Here's how the part is built. I have some questions about the finished solid (model axes, mm). A direction names the side the tool comes from. Round coordinates to 2 decimals unless told otherwise and drop trailing zeros. Write each loop counter-clockwise with the first axis right and the second up, starting at its lowest first coordinate (ties: lowest second). Pieces come first, ordered by that corner, then holes. Notation, with made-up numbers: (-5.5, -11.5) -> (22.5, -11.5) arc R21 cw to (22.5, 3.5) -> close; hole circle Ø4 at (89, -30.75). An arc over 180 degrees is marked (long way). Put each result on its own line as item: value. Start each with the question number.
1) I want a section at A-A, the plane y = 2.4. List the corners of the cut face in (x, z) for me.
2) Will these pins go through, and if not, where does the flat tip stop? P1, Ø0.6, axis at x = 1.5, z = -2, coming from the +Y side; P2, Ø1.4, axis at y = 1.5, z = -3, coming from the -X side; P3, Ø0.9, axis at x = -1.5, z = -6.1, coming from the -Y side; P4, Ø1.7, axis at x = -1.5, z = -2.1, coming from the -Y side.
3) If I drill on line 1 along Z through (x, y) = (-1.5, 1.05); line 2 along X through (y, z) = (1.2, -2.5); line 3 along X through (y, z) = (1.25, -2.75), over which ranges is the centre line in solid material (lowest first)? Write a range as [from, to].
4) I want a section at C-C, the plane z = -6.5. List the corners of the cut face in (x, y) for me, then the cut area to 3 significant figures.
5) I want a section at B-B, the plane x = 0.75. List the corners of the cut face in (y, z) for me.
6) We'd pull the mould along X, two halves only. Please class faces 4 (the flat face through (1, 1.65, -2)), 5 (the flat face through (-6.2, 1, -4)), 6 (the flat face through (-7.53, 1.37, -3.97)): released by +X, released by -X, zero draft, split by the parting line, or undercut.
7) Which directions (+Z, -Z, +X, -X, +Y, -Y) give clear straight access to the entire face, cutting with the end or side of a thin tool? Please do faces 1 (the flat face through (-4, 0, -4)), 2 (the flat face through (1, 1.05, -2)), 3 (the flat face through (-6.764, 1.369, -4.287)).
8) I want a section at D-D, the plane y = 1.35. List the corners of the cut face in (x, z) for me.
Autodesk Inventor part; units mm, degrees
ref_plane "YZ Plane" through (0, 0, 0) normal (1, 0, 0) x (0, 1, 0)
ref_plane "XZ Plane" through (0, 0, 0) normal (0, 1, 0) x (-1, 0, 0)
ref_plane "XY Plane" through (0, 0, 0) normal (0, 0, 1) x (1, 0, 0)
sketch "Sketch1" plane through (0, 0, 0) normal (0, 1, 0) x (-1, 0, 0)
  line L0 (0, 0) -> (6.2, 0)
  line L1 (6.2, 0) -> (6.2, -8.2)
  line L2 (6.2, -8.2) -> (0, -8.2)
  line L3 (0, -8.2) -> (0, 0)
  dimension "d0" = 8.2
  dimension "d1" = 6.2
extrude "Extrusion1" add sketch "Sketch1" along normal blind 2.7
sketch "Sketch2" plane through (0, 2.7, 0) normal (0, 1, 0) x (1, 0, 0)
  line L0 (-6.2, 8.2) -> (-6.2, 0)
  line L1 (-6.2, 0) -> (0, 0)
  line L2 (0, 0) -> (0, 8.2)
  line L3 (0, 8.2) -> (-6.2, 8.2)
  line L4 (-6.2, 8.2) -> (-6.2, 0)
  line L5 (-6.2, 0) -> (-7.2442, 7.9316)
  line L6 (-7.2442, 7.9316) -> (-8.0374, 7.8271)
  line L7 (-8.0374, 7.8271) -> (-7.0069, 0)
  line L8 (-6.2, 0) -> (-7.0069, 0)
  dimension "d4" = 8
  dimension "d5" = 7.5
  dimension "d6" = 0.8
extrude "Extrusion2" add sketch "Sketch2" against normal up to surface (2.7 mm away) contours L8 L7 L6 L5
sketch "Sketch3" plane through (0, 0, 0) normal (0, -1, 0) x (1, 0, 0)
  line L0 (-6.2, -8.2) -> (-6.2, 0)
  line L1 (0, -8.2) -> (-6.2, -8.2)
  line L2 (0, 0) -> (0, -8.2)
  line L3 (-6.2, 0) -> (0, 0)
  line L4 (-7.0069, 0) -> (-8.0374, -7.8271)
  line L5 (-8.0374, -7.8271) -> (-7.2442, -7.9316)
  line L6 (-7.2442, -7.9316) -> (-6.2, 0)
  line L7 (-6.2, 0) -> (-7.0069, 0)
  line L8 (-6.2, 0) -> (0, 0)
  circle A0 centre (-6.2, 0) radius 0.75
  point P0 (-6.2979, -0.7436)
  point P1 (-6.2, -0.75)
  dimension "d9" = 1.5
extrude "Extrusion3" add sketch "Sketch3" against normal up to surface (2.7 mm away) contours A0 L6 L0
sketch "Sketch4" plane through (0, 2.7, 0) normal (0, 1, 0) x (1, 0, 0)
  line L0 (-6.2, 8.2) -> (-6.2, 0.75)
  arc A0 (-6.2, 0.75) -> (-6.2979, 0.7436) centre (-6.2, 0) ccw
  line L1 (-6.2979, 0.7436) -> (-7.2442, 7.9316)
  line L2 (-7.2442, 7.9316) -> (-8.0374, 7.8271)
  line L3 (-8.0374, 7.8271) -> (-7.0069, 0)
  line L4 (-7.0069, 0) -> (0, 0)
  line L5 (0, 0) -> (0, 8.2)
  line L6 (0, 8.2) -> (-6.2, 8.2)
  line L7 (0, 0) -> (0, 8.2)
  line L8 (0, 4.1) -> (-1.5, 4.1)
  line L9 (-1.5, 4.1) -> (-1.5, 6.1)
  line L10 (-1.5, 4.1) -> (-1.5, 2.1)
  circle A1 centre (-1.5, 2.1) radius 0.75
  circle A2 centre (-1.5, 6.1) radius 0.75
  dimension "d12" = 1.5
  dimension "d13" = 2
  dimension "d14" = 2
  dimension "d15" = 1.5
  dimension "d16" = 1.5
extrude "Extrusion4" cut sketch "Sketch4" against normal blind 2.7 contours A1 | A2
sketch "Sketch5" plane through (0, 0, 0) normal (1, 0, 0) x (0, 0, -1)
  line L0 (0, 0) -> (8.2, 0)
  line L1 (8.2, 0) -> (8.2, 2.7)
  line L2 (0, 2.7) -> (8.2, 2.7)
  line L3 (0, 0) -> (0, 2.7)
  line L4 (0.7436, 2.7) -> (7.9316, 2.7)
  line L5 (4.1, 2.7) -> (4.1, 1.35)
  line L6 (7.9316, 0) -> (0.7436, 0)
  line L7 (3.7, 1.35) -> (4.5, 1.35) construction
  line L8 (3.7, 1.05) -> (4.5, 1.05)
  line L9 (4.5, 1.65) -> (3.7, 1.65)
  arc A0 (3.7, 1.65) -> (3.7, 1.05) centre (3.7, 1.35) ccw
  arc A1 (4.5, 1.05) -> (4.5, 1.65) centre (4.5, 1.35) ccw
  line L10 (4.1, 1.35) -> (6.4, 1.35)
  line L11 (6, 1.35) -> (6.8, 1.35) construction
  line L12 (6, 1.05) -> (6.8, 1.05)
  line L13 (6.8, 1.65) -> (6, 1.65)
  arc A2 (6, 1.65) -> (6, 1.05) centre (6, 1.35) ccw
  arc A3 (6.8, 1.05) -> (6.8, 1.65) centre (6.8, 1.35) ccw
  line L14 (4.1, 1.35) -> (1.8, 1.35)
  line L15 (1.4, 1.35) -> (2.2, 1.35) construction
  line L16 (1.4, 1.05) -> (2.2, 1.05)
  line L17 (2.2, 1.65) -> (1.4, 1.65)
  arc A4 (1.4, 1.65) -> (1.4, 1.05) centre (1.4, 1.35) ccw
  arc A5 (2.2, 1.05) -> (2.2, 1.65) centre (2.2, 1.35) ccw
  dimension "d19" = 1.35
  dimension "d20" = 0.4
  dimension "d21" = 0.6
  dimension "d22" = 2.3
  dimension "d23" = 0.4
  dimension "d24" = 0.6
  dimension "d25" = 2.3
  dimension "d26" = 0.4
  dimension "d27" = 0.6
extrude "Extrusion5" add sketch "Sketch5" along normal blind 3 contours A2 L13 A3 L12 | A5 L16 A4 L17 | L9 A1 L10 L5 | L5 L14 A0 L9 | L10 A1 L8 A0 L14
properties part number "micro_switch_1"
Findings:
1. outline: (-8.04, -7.83) -> (-7.24, -7.93) -> (-6.3, -0.74) arc R0.75 ccw to (-6.2, -0.75) -> (-6.2, -8.2) -> (0, -8.2) -> (0, 0) -> (-7.01, 0) -> close; hole circle Ø1.5 at (-1.5, -6.1); hole circle Ø1.5 at (-1.5, -2.1)
2. P1: stops at y = 1.65
2. P2: stops at x = -7.49
2. P3: passes through
2. P4: stops at y = 0
3. line 1: z = [-8.2, -6.85], [-5.35, -2.85], [-1.35, 0]
3. line 2: x = [-7.34, -6.53], [-6.2, -2.13], [-0.87, 0]
3. line 3: x = [-7.37, -6.56], [-6.2, -1.87], [-1.13, 0]
4. outline: (-7.86, 0) -> (-7.06, 0) -> (-7.06, 2.7) -> (-7.86, 2.7) -> close; (-6.2, 0) -> (-2.13, 0) -> (-2.13, 2.7) -> (-6.2, 2.7) -> close; (-0.87, 0) -> (0, 0) -> (0, 1.05) -> (3, 1.05) -> (3, 1.65) -> (0, 1.65) -> (0, 2.7) -> (-0.87, 2.7) -> close
4. area: 17.3 mm2
5. outline: (1.05, -6.8) arc R0.3 ccw to (1.65, -6.8) -> (1.65, -6) arc R0.3 ccw to (1.05, -6) -> close; (1.05, -4.5) arc R0.3 ccw to (1.65, -4.5) -> (1.65, -3.7) arc R0.3 ccw to (1.05, -3.7) -> close; (1.05, -2.2) arc R0.3 ccw to (1.65, -2.2) -> (1.65, -1.4) arc R0.3 ccw to (1.05, -1.4) -> close
6. face 4: zero draft
6. face 5: undercut
6. face 6: released by -X
7. face 1: +Z, -Z, +X, -X, -Y
7. face 2: +Z, -Z, +X, -Y
7. face 3: -Z, +Y, -Y
8. outline: (-8.04, -7.83) -> (-7.24, -7.93) -> (-6.3, -0.74) arc R0.75 ccw to (-6.2, -0.75) -> (-6.2, -8.2) -> (0, -8.2) -> (0, -7.1) -> (3, -7.1) -> (3, -5.7) -> (0, -5.7) -> (0, -4.8) -> (3, -4.8) -> (3, -3.4) -> (0, -3.4) -> (0, -2.5) -> (3, -2.5) -> (3, -1.1) -> (0, -1.1) -> (0, 0) -> (-7.01, 0) -> close; hole circle Ø1.5 at (-1.5, -6.1); hole circle Ø1.5 at (-1.5, -2.1)
